from build123d import *

# Parameters (mm, degrees)
SKETCH014_R             = 1.5
POCKET_DEPTH            = 271.834281
POLARPATTERN_COUNT      = 6
PAD_DEPTH               = 40
SKETCH016_W             = 21.623292
SKETCH016_H             = 27.433631
POCKET001_DEPTH         = 35
BODY003_PLACEMENT_ANGLE = 90


with BuildPart() as part:
    # Sketch → Revolution (revolve)
    with BuildSketch(Plane.XZ):
        Polygon((14, 0), (14, 5), (26.5, 5), (26.5, 40), (45, 40), (45, 0), align=None)
    revolve(axis=Axis((0, 0, 0), (0, 0, 1)))

    # Sketch014 → Pocket (cut, through all)
    with BuildSketch(Plane.XY.offset(5)):
        with Locations((0, 19)):
            Circle(SKETCH014_R)
    pocket = extrude(amount=-POCKET_DEPTH, mode=Mode.SUBTRACT)

    # PolarPattern: Pocket ×6 about axis
    polarpattern_axis = Axis((0, 0, 5), (0, 0, 1))
    for i in range(1, POLARPATTERN_COUNT):
        add(pocket.rotate(polarpattern_axis, i * 360 / POLARPATTERN_COUNT), mode=Mode.SUBTRACT)

    # Sketch015 (on Face12 of PolarPattern) → Pad (join)
    with BuildSketch(Plane(origin=(0, 0, 40), x_dir=(-1, 0, 0), z_dir=(0, 0, 1))):
        with BuildLine():
            Line((-27, 51), (-27, 36))
            ThreePointArc((-21.35998, 39.607465), (-24.247172, 37.908767), (-27, 36))
            Line((-21.35998, 39.607465), (21.35998, 39.607465))
            ThreePointArc((27, 36), (24.247172, 37.908767), (21.35998, 39.607465))
            Line((27, 36), (27, 51))
            Line((27, 51), (-27, 51))
        make_face()
    extrude(amount=-PAD_DEPTH)

    # Sketch016 (on Face2 of Pad) → Pocket001 (cut)
    with BuildSketch(Plane.XZ.offset(51)):
        with Locations((0, 27.158627)):
            Rectangle(SKETCH016_W, SKETCH016_H)
    extrude(amount=-POCKET001_DEPTH, mode=Mode.SUBTRACT)


with BuildPart() as part_1:
    # Body003 placement: moved
    add(part.part.moved(Location((0, 0, 22))).rotate(Axis((0, 0, 22), (0, 0, 1)), BODY003_PLACEMENT_ANGLE))


solid = part_1.part
Can you work these out from the model? Positions are in its coordinate system, mm. A direction names the side the tool comes from. Round coordinates to 2 decimals unless told otherwise and drop trailing zeros. Loops run counter-clockwise (first coordinate to the right, second up) from the corner with the lowest first, then second, coordinate; pieces in that order, holes last. Notation, with made-up numbers: (49, 46.5) - (101, 46.5) arc R17 cw to (101, 63.5) - close; hole circle Ø11 at (-33.5, -7.75). An arc over 180 degrees is marked (long way). Write item = value, one per line. Start each with the question number.
(1) If we section it at B-B (y = 0): Please give me the cut outline in (x, z).
(2) If we section it at C-C (z = 41): Please give me the cut outline in (x, y).
(3) If we section it at A-A (x = 0): Please give me the cut outline in (y, z), and give its area (4 significant figures).
(4) If I drill on probe 1 along X at (y, z) = (0, 24.65); probe 2 along Y at (x, z) = (46, 40); probe 3 along Y at (x, z) = (-9.5, 23.1), over which ranges is the centre line in solid material (lowest first)? Write a range as [from, to].
(5) If we section it at D-D (x = 32.5): Please give me the cut outline in (y, z), and give its area (3 significant figures).
(6) For P1, Ø1.8, axis at x = 9.5, y = 16.45, coming from the +Z side; P2, Ø4, axis at x = -9.5, y = 16.45, coming from the -Z side; P3, Ø5, axis at x = -9.5, y = -16.45, coming from the +Z side; P4, Ø10, axis at x = -21.5, z = 29.5, coming from the +Y side, each with a flat end and sliding along its axis, tell me the tip position at first contact or that it passes through.
(7) For faces 1 (the face through (11, -11, 27)), 2 (the face through (44, 27, 42)), 3 (the face through (38, 0, 35.442)), which set-ups out of +Z, -Z, +X, -X, +Y, -Y let a thin tool reach every point of the face, with its end or its side?
Ans:
q1.outline = (-45, 22) - (-20.5, 22) - (-20.5, 27) - (-26.5, 27) - (-26.5, 62) - (-45, 62) - close; (-17.5, 22) - (-14, 22) - (-14, 27) - (-17.5, 27) - close; (14, 22) - (17.5, 22) - (17.5, 27) - (14, 27) - close; (20.5, 22) - (51, 22) - (51, 35.44) - (26.5, 35.44) - (26.5, 27) - (20.5, 27) - close
q2.outline = (24.19, -10.81) arc R26.5 cw (long way) to (24.19, 10.81) - (51, 10.81) - (51, 27) - (36, 27) arc R45 ccw (long way) to (36, -27) - (51, -27) - (51, -10.81) - close
q3.outline = (-45, 22) - (-14, 22) - (-14, 27) - (-26.5, 27) - (-26.5, 62) - (-45, 62) - close; (14, 22) - (45, 22) - (45, 62) - (26.5, 62) - (26.5, 27) - (14, 27) - close
q3.area = 1,605 mm²
q4.probe_1 = [-45, -20.5], [-17.5, -14], [14, 17.5], [20.5, 51]
q4.probe_2 = [-27, -10.81], [10.81, 27]
q4.probe_3 = [-43.99, -17.95], [-14.95, -10.28], [10.28, 14.95], [17.95, 43.99]
q5.outline = (-31.12, 22) - (31.12, 22) - (31.12, 62) - (10.81, 62) - (10.81, 35.44) - (-10.81, 35.44) - (-10.81, 62) - (-31.12, 62) - close
q5.area = 1,920 mm²
q6.P1 = through
q6.P2 = 22
q6.P3 = 27
q6.P4 = 41.87
q7.face_1 = +Z
q7.face_2 = +Z, -Z, +X, +Y
q7.face_3 = +Z, +X
